Geometry check sheet. Reference: drawing and pictorial views, mm from the part's lowest x, y, z. A direction names the side the tool comes from. Coordinates: 2 decimals unless noted, no trailing zeros. Write each loop counter-clockwise with the first axis right and the second up, starting at its lowest first coordinate (ties: lowest second). Pieces come first, ordered by that corner, then holes. Notation, with made-up numbers: M 8.25,82 L 63.25,82 A27 ccw 63.25,99 Z; hole C 44.25,68 d2. An arc over 180 degrees is marked long. One line per item, written item: value.
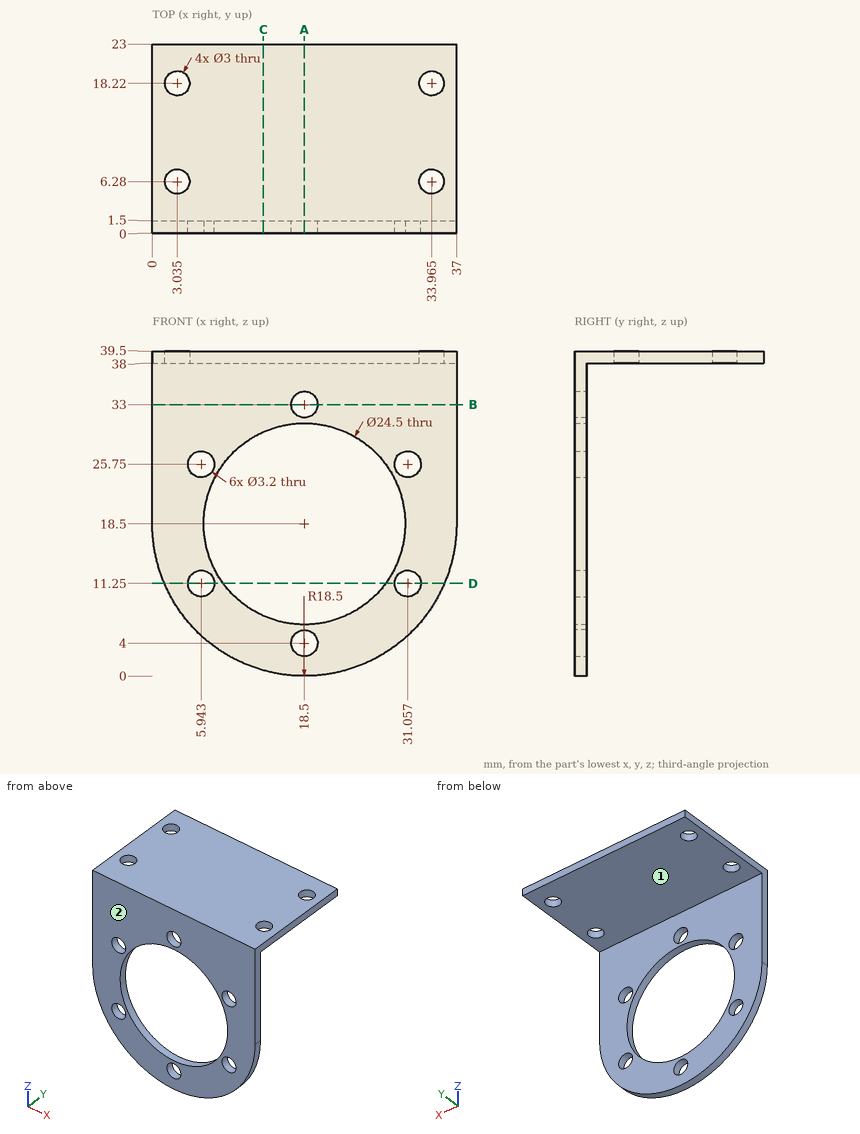
Item 1: Cross-section at D-D, the plane z = 11.25. Enter the section's corners in (x, y).
The answers:
outline: M 1.48,0 L 4.34,0 L 4.34,1.5 L 1.48,1.5 Z; M 7.54,0 L 8.63,0 L 8.63,1.5 L 7.54,1.5 Z; M 28.37,0 L 29.46,0 L 29.46,1.5 L 28.37,1.5 Z; M 32.66,0 L 35.52,0 L 35.52,1.5 L 32.66,1.5 Z
Item 2: Go/stop test with flat-tipped pins: P1, Ø4, axis at x = 3.04, y = 6.28, coming from the -Z side; P2, Ø4, axis at x = 18.5, z = 4, coming from the +Y side. Record where each tip stops, or that it passes through.
The answers:
P1: stops at z = 38
P2: stops at y = 1.5
Item 3: Access from +Z, -Z, +X, -X, +Y, -Y to the whole of each face (thin tool, end or side, straight path). Record for the marked faces 1 and 2.
The answers:
face 1: -Z, +X, -X, +Y
face 2: +Z, -Z, +X, -X, -Y
Item 4: Cross-section at A-A, the plane x = 18.5. Enter the section's corners in (y, z).
The answers:
outline: M 0,0 L 1.5,0 L 1.5,2.4 L 0,2.4 Z; M 0,5.6 L 1.5,5.6 L 1.5,6.25 L 0,6.25 Z; M 0,30.75 L 1.5,30.75 L 1.5,31.4 L 0,31.4 Z; M 0,34.6 L 1.5,34.6 L 1.5,38 L 23,38 L 23,39.5 L 0,39.5 Z
Item 5: Cross-section at B-B, the plane z = 33. Enter the section's corners in (x, y).
The answers:
outline: M 0,0 L 16.9,0 L 16.9,1.5 L 0,1.5 Z; M 20.1,0 L 37,0 L 37,1.5 L 20.1,1.5 Z
Item 6: Scan lines: line 1 (X direction, y = 1.2, z = 11.25) (1 decimal); line 2 (X direction, y = 1.2, z = 18.5); line 3 (Y direction, x = 21, z = 31). Record each from-to range of solid material in increasing order.
The answers:
line 1: x = 1.5 to 4.3, 7.5 to 8.6, 28.4 to 29.5, 32.7 to 35.5
line 2: x = 0 to 6.25, 30.75 to 37
line 3: y = 0 to 1.5
Item 7: Cross-section at C-C, the plane x = 13.5. Enter the section's corners in (y, z).
The answers:
outline: M 0,0.69 L 1.5,0.69 L 1.5,7.32 L 0,7.32 Z; M 0,29.68 L 1.5,29.68 L 1.5,38 L 23,38 L 23,39.5 L 0,39.5 Z
